The listing builds one solid part. Answer for the finished solid, in the listing's coordinates (mm). Face numbers are marked on the shaded views. Round coordinates to 2 decimals unless told otherwise and drop trailing zeros. Write each loop counter-clockwise with the first axis right and the second up, starting at its lowest first coordinate (ties: lowest second). Pieces come first, ordered by that corner, then holes. Notation, with made-up numbers: (18.5, 46.5) - (26.5, 46.5) arc R10 cw to (26.5, 54.5) - close; hole circle Ø9 at (-36.5, -33.5). An arc over 180 degrees is marked (long way). Return JSON: item names as keys, results as strings. Group by question number.
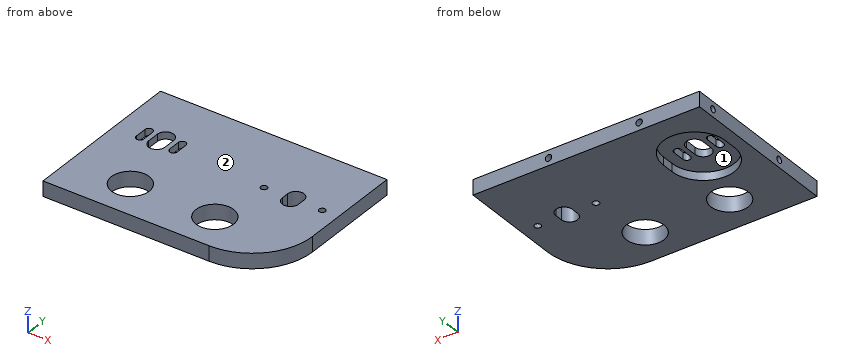
from build123d import *

# Parameters (mm, degrees)
SKETCH1_W                 = 95.287460045
SKETCH1_H                 = 69.153467802
SKETCH1_R                 = 7.9375
BOSS_EXTRUDE1_DEPTH       = 6.35
FILLET1_R                 = 25.4
F_6_32_TAPPED_HOLE1_D     = 2.7051
F_6_32_TAPPED_HOLE1_DEPTH = 10.9728
F_6_32_TAPPED_HOLE1_TIP   = 0.81269403
CUT_EXTRUDE2_DEPTH        = 82.189684793
CUT_EXTRUDE1_DEPTH        = 3.367
F_6_32_TAPPED_HOLE2_D     = 2.7051
F_6_32_TAPPED_HOLE2_DEPTH = 9.398
F_6_32_TAPPED_HOLE2_TIP   = 0.81269403
F_6_32_TAPPED_HOLE3_D     = 2.7051
F_6_32_TAPPED_HOLE3_DEPTH = 9.398
F_6_32_TAPPED_HOLE3_TIP   = 0.81269403


with BuildPart() as part:
    # Sketch1 → Boss-Extrude1 (new body)
    with BuildSketch(Plane.XY.offset(-6.35)):
        with Locations((-13.289407805, 18.701733901)):
            Rectangle(SKETCH1_W, SKETCH1_H)
        with Locations((-35.533137827, 0)):
            Circle(SKETCH1_R, mode=Mode.SUBTRACT)
        Circle(SKETCH1_R, mode=Mode.SUBTRACT)
        with BuildLine():
            Line((11.875322218, 23.115967802), (11.875322218, 26.290967802))
            ThreePointArc((11.875322218, 26.290967802), (15.304322218, 29.719967802), (18.733322218, 26.290967802))
            Line((18.733322218, 26.290967802), (18.733322218, 23.115967802))
            ThreePointArc((18.733322218, 23.115967802), (15.304322218, 19.686967802), (11.875322218, 23.115967802))
        make_face(mode=Mode.SUBTRACT)
    extrude(amount=BOSS_EXTRUDE1_DEPTH)

    # Fillet1
    fillet1_edges = [part.edges().sort_by_distance(p)[0] for p in [
        (34.354322218, -15.875, -3.175),
    ]]
    fillet(fillet1_edges, radius=FILLET1_R)

    # #6-32 Tapped Hole1
    with Locations(Plane(origin=(0, 0, -6.35), x_dir=(-1, 0, 0), z_dir=(0, 0, -1))):
        with Locations((-27.559822218, 24.703467802), (-3.048822218, 24.703467802)):
            Hole(F_6_32_TAPPED_HOLE1_D / 2, depth=F_6_32_TAPPED_HOLE1_DEPTH)
            with Locations((0, 0, -(F_6_32_TAPPED_HOLE1_DEPTH + F_6_32_TAPPED_HOLE1_TIP / 2))):  # 118° drill point
                Cone(0, F_6_32_TAPPED_HOLE1_D / 2, F_6_32_TAPPED_HOLE1_TIP, mode=Mode.SUBTRACT)

    # Sketch4<3> → Cut-Extrude2 (cut, through all)
    with BuildSketch(Plane(origin=(0, 0, -6.35), x_dir=(-1, 0, 0), z_dir=(0, 0, -1))):
        with BuildLine():
            Line((39.282270444, 30.74802952), (39.282270444, 25.573029456))
            ThreePointArc((39.282270444, 25.573029456), (42.707270452, 22.148029448), (46.13227046, 25.573029456))
            Line((46.13227046, 25.573029456), (46.13227046, 30.74802952))
            ThreePointArc((46.13227046, 30.74802952), (42.707270452, 34.173029528), (39.282270444, 30.74802952))
        make_face()
        with BuildLine():
            Line((48.119770452, 30.74802952), (48.119770452, 25.573029456))
            ThreePointArc((48.119770452, 25.573029456), (49.707270452, 23.985529456), (51.294770452, 25.573029456))
            Line((51.294770452, 25.573029456), (51.294770452, 30.74802952))
            ThreePointArc((51.294770452, 30.74802952), (49.707270452, 32.33552952), (48.119770452, 30.74802952))
        make_face()
        with BuildLine():
            Line((37.294770452, 30.74802952), (37.294770452, 25.573029456))
            ThreePointArc((37.294770452, 25.573029456), (35.707270452, 23.985529456), (34.119770452, 25.573029456))
            Line((34.119770452, 25.573029456), (34.119770452, 30.74802952))
            ThreePointArc((34.119770452, 30.74802952), (35.707270452, 32.33552952), (37.294770452, 30.74802952))
        make_face()
    extrude(amount=-CUT_EXTRUDE2_DEPTH, mode=Mode.SUBTRACT)

    # Sketch4 → Cut-Extrude1 (cut)
    with BuildSketch(Plane(origin=(0, 0, -6.35), x_dir=(-1, 0, 0), z_dir=(0, 0, -1))):
        with BuildLine():
            Line((29.607270452, 30.74802952), (29.607270452, 25.573029456))
            ThreePointArc((29.607270452, 25.573029456), (42.707270452, 12.473029456), (55.807270452, 25.573029456))
            Line((55.807270452, 25.573029456), (55.807270452, 30.74802952))
            ThreePointArc((55.807270452, 30.74802952), (42.707270452, 43.84802952), (29.607270452, 30.74802952))
        make_face()
        with BuildLine():
            Line((46.13227046, 30.74802952), (46.13227046, 25.573029456))
            ThreePointArc((46.13227046, 25.573029456), (42.707270452, 22.148029448), (39.282270444, 25.573029456))
            Line((39.282270444, 25.573029456), (39.282270444, 30.74802952))
            ThreePointArc((39.282270444, 30.74802952), (42.707270452, 34.173029528), (46.13227046, 30.74802952))
        make_face(mode=Mode.SUBTRACT)
        with BuildLine():
            Line((34.119770452, 30.74802952), (34.119770452, 25.573029456))
            ThreePointArc((34.119770452, 25.573029456), (35.707270452, 23.985529456), (37.294770452, 25.573029456))
            Line((37.294770452, 25.573029456), (37.294770452, 30.74802952))
            ThreePointArc((37.294770452, 30.74802952), (35.707270452, 32.33552952), (34.119770452, 30.74802952))
        make_face(mode=Mode.SUBTRACT)
        with BuildLine():
            Line((48.119770452, 30.74802952), (48.119770452, 25.573029456))
            ThreePointArc((48.119770452, 25.573029456), (49.707270452, 23.985529456), (51.294770452, 25.573029456))
            Line((51.294770452, 25.573029456), (51.294770452, 30.74802952))
            ThreePointArc((51.294770452, 30.74802952), (49.707270452, 32.33552952), (48.119770452, 30.74802952))
        make_face(mode=Mode.SUBTRACT)
    extrude(amount=-CUT_EXTRUDE1_DEPTH, mode=Mode.SUBTRACT)

    # #6-32 Tapped Hole2
    with Locations(Plane(origin=(0, 53.278467802, 0), x_dir=(1, 0, 0), z_dir=(0, 1, 0))):
        with Locations((-35.533137827, 3.175), (2.604322218, 3.175)):
            Hole(F_6_32_TAPPED_HOLE2_D / 2, depth=F_6_32_TAPPED_HOLE2_DEPTH)
            with Locations((0, 0, -(F_6_32_TAPPED_HOLE2_DEPTH + F_6_32_TAPPED_HOLE2_TIP / 2))):  # 118° drill point
                Cone(0, F_6_32_TAPPED_HOLE2_D / 2, F_6_32_TAPPED_HOLE2_TIP, mode=Mode.SUBTRACT)

    # #6-32 Tapped Hole3
    with Locations(Plane.ZY.offset(60.933137827)):
        with Locations((-3.175, 6.35), (-3.175, 45.340967802)):
            Hole(F_6_32_TAPPED_HOLE3_D / 2, depth=F_6_32_TAPPED_HOLE3_DEPTH)
            with Locations((0, 0, -(F_6_32_TAPPED_HOLE3_DEPTH + F_6_32_TAPPED_HOLE3_TIP / 2))):  # 118° drill point
                Cone(0, F_6_32_TAPPED_HOLE3_D / 2, F_6_32_TAPPED_HOLE3_TIP, mode=Mode.SUBTRACT)


solid = part.part
(1) Flat-ended cylindrical pins translate along their axes: pin 1 (21 mm diameter, centred on x = -45, y = 31.5, fed in from -Z); pin 2 (2.5 mm diameter, centred on y = 45.34, z = -3.18, fed in from -X). Find the tip coordinate at first contact, or state that the pin passes through.
(2) Determine the mould class of the marked faces 1 and 2 for opening direction X: +X half, -X half, draft (parallel to the pull), parting line (faces both ways), or undercut.
(3) Find section C-C (y = 27.5). Write down the section's boundary in (x, z).
(4) Find section B-B (y = 0). Write down the section's boundary in (x, z), plus the area to 3 significant figures.
(5) Find section D-D (y = 48). Write down the section's boundary in (x, z) (3 decimals).
(6) Consider line 1 (Y direction, x = 0, z = -1.75) (1 decimal); line 2 (Y direction, x = -40, z = -0.25) (3 decimals); line 3 (Y direction, x = -41, z = -5) (3 decimals). Determine where each line is inside the solid, lowest interval first.
Check sheet entries:
{
 "1": {"pin 1": "stops at z = -2.98", "pin 2": "stops at x = -51.48"},
 "2": {"face 1": "undercut", "face 2": "draft"},
 "3": {"outline": "(-60.93, -6.35) - (-55.81, -6.35) - (-55.81, -2.98) - (-51.29, -2.98) - (-51.29, 0) - (-60.93, 0) - close; (-48.12, -2.98) - (-46.13, -2.98) - (-46.13, 0) - (-48.12, 0) - close; (-39.28, -2.98) - (-37.29, -2.98) - (-37.29, 0) - (-39.28, 0) - close; (-34.12, -2.98) - (-29.61, -2.98) - (-29.61, -6.35) - (12.1, -6.35) - (12.1, 0) - (-34.12, 0) - close; (18.51, -6.35) - (34.35, -6.35) - (34.35, 0) - (18.51, 0) - close"},
 "4": {"outline": "(-60.93, -6.35) - (-43.47, -6.35) - (-43.47, 0) - (-60.93, 0) - close; (-27.6, -6.35) - (-7.94, -6.35) - (-7.94, 0) - (-27.6, 0) - close; (7.94, -6.35) - (32.5, -6.35) - (32.5, 0) - (7.94, 0) - close", "area": "392 mm^2"},
 "5": {"outline": "(-60.933, -6.35) - (34.354, -6.35) - (34.354, 0) - (-60.933, 0) - close; hole circle Ø2.705 at (-35.533, -3.175); hole circle Ø2.705 at (2.604, -3.175)"},
 "6": {"line 1": "y = -15.9 to -7.9, 7.9 to 53.3", "line 2": "y = -15.875 to -6.561, 6.561 to 23.475, 32.846 to 53.278", "line 3": "y = -15.875 to -5.755, 5.755 to 12.585, 43.736 to 53.278"}
}
